Can you work these out from the model? Positions are in its coordinate system, mm. A direction names the side the tool comes from. Coordinates: 2 decimals unless noted, no trailing zeros. Write each loop counter-clockwise with the first axis right and the second up, starting at its lowest first coordinate (ties: lowest second). Pieces come first, ordered by that corner, then holes. Notation, with made-up numbers: (47.5, -28) - (102.5, -28) arc R17 cw to (102.5, 2) - close; hole circle Ø1 at (34.25, -19). An arc over 180 degrees is marked (long way). One line per question, with ' | ' between items. Start each with the question number.
from build123d import *

# Parameters (mm, degrees)
SKETCH_1_W          = 80
SKETCH_1_H          = 25
EXTRUDE_1_DEPTH     = 8
EXTRUDE_2_DEPTH     = 1.7
SKETCH_5_W          = 2.2
SKETCH_5_H          = 1.7
CUT_EXTRUDE_1_DEPTH = 7
SKETCH_3_R          = 1.35
CUT_EXTRUDE_2_DEPTH = 85.374699999


with BuildPart() as part:
    # 草图1 → 凸台-拉伸1 (new body)
    with BuildSketch(Plane.XY):
        with Locations((40, -12.5)):
            Rectangle(SKETCH_1_W, SKETCH_1_H)
    extrude(amount=EXTRUDE_1_DEPTH)

    # 草图2 → 凸台-拉伸2 (add)
    with BuildSketch(Plane(origin=(0, 0, 0), x_dir=(-1, 0, 0), z_dir=(0, 0, -1))):
        with BuildLine():
            Line((-68, -10.85), (-12.5, -10.85))
            ThreePointArc((-12.5, -10.85), (-10.85, -12.5), (-12.5, -14.15))
            Line((-12.5, -14.15), (-68, -14.15))
            ThreePointArc((-68, -14.15), (-69.65, -12.5), (-68, -10.85))
        make_face()
    extrude(amount=EXTRUDE_2_DEPTH)

    # 草图5 → 切除-拉伸1 (cut)
    with BuildSketch(Plane.XZ.offset(14.15)):
        with Locations((40.2, -0.85)):
            Rectangle(SKETCH_5_W, SKETCH_5_H)
    extrude(amount=-CUT_EXTRUDE_1_DEPTH, mode=Mode.SUBTRACT)

    # 草图3 → 切除-拉伸2 (cut, through all)
    with BuildSketch(Plane(origin=(0, 0, -1.7), x_dir=(-1, 0, 0), z_dir=(0, 0, -1))):
        with Locations((-68, -12.5)):
            Circle(SKETCH_3_R)
        with Locations((-12.5, -12.5)):
            Circle(SKETCH_3_R)
    extrude(amount=-CUT_EXTRUDE_2_DEPTH, mode=Mode.SUBTRACT)


solid = part.part
(1) I'm going to push flat-ended pins straight in: pin 1 (12 mm diameter, centred on x = 27, y = -21, fed in from -Z); pin 2 (1.4 mm diameter, centred on y = -12.5, z = -1, fed in from -X); pin 3 (1.4 mm diameter, centred on x = 21, z = -1, fed in from -Y); pin 4 (8 mm diameter, centred on x = 36.5, y = -10.5, fed in from -Z). Where does each tip first touch, or does it pass through?
(2) If we section it at D-D on x = 8.5: List the corners of the cut face in (y, z) for me.
(3) If we mould it in two halves opening along X, with no side actions, what happens to faces 4 (the face through (26, -10.85, -1)), 5 (the face through (80, -13, 4)), 6 (the face through (12.676, -11.161, 3.082))? For each: +X half, -X half, draft (parallel to the pull), parting line (faces both ways), or undercut.
(4) If we section it at B-B on x = 47.5: List the corners of the cut face in (y, z) for me.
(5) If we section it at C-C on y = -21.75: List the corners of the cut face in (x, z) for me.
(6) If I drill on probe 1 along Z at (x, y) = (9, -4.75); probe 2 along Y at (x, z) = (69, -1); probe 3 along Y at (x, z) = (69.5, -0.25), over which ranges is the centre line in solid material (lowest first)?
(7) If we section it at A-A on y = -12.5: List the corners of the cut face in (x, z) for me, plus the area to 3 significant figures.
(8) Which directions (+Z, -Z, +X, -X, +Y, -Y) give clear straight access to the entire face, cutting with the end or side of a thin tool? Please do faces 1 (the face through (26, -14.15, -1)), 2 (the face through (39.1, -13, -1)), 3 (the face through (55, -10.85, -1)).
Values:
1) pin 1: z = 0 | pin 2: x = 10.85 | pin 3: y = -14.15 | pin 4: z = -1.7
2) outline: (-25, 0) - (0, 0) - (0, 8) - (-25, 8) - close
3) face 4: draft | face 5: +X half | face 6: undercut
4) outline: (-25, 0) - (-14.15, 0) - (-14.15, -1.7) - (-10.85, -1.7) - (-10.85, 0) - (0, 0) - (0, 8) - (-25, 8) - close
5) outline: (0, 0) - (80, 0) - (80, 8) - (0, 8) - close
6) probe 1: 0 to 8 | probe 2: -13.81 to -13.41, -11.59 to -11.19 | probe 3: -13.19 to -11.81
7) outline: (0, 0) - (10.85, 0) - (10.85, -1.7) - (11.15, -1.7) - (11.15, 8) - (0, 8) - close; (13.85, -1.7) - (39.1, -1.7) - (39.1, 0) - (41.3, 0) - (41.3, -1.7) - (66.65, -1.7) - (66.65, 8) - (13.85, 8) - close; (69.35, -1.7) - (69.65, -1.7) - (69.65, 0) - (80, 0) - (80, 8) - (69.35, 8) - close | area: 684 mm2
8) face 1: -Z, +X, -X, -Y | face 2: -Z, +Y, -Y | face 3: -Z, +X, -X, +Y
